Here's how the part is built. I have some questions about the finished solid (model axes, mm). A direction names the side the tool comes from. Round coordinates to 2 decimals unless told otherwise and drop trailing zeros. Order: outer loops, then holes, each group sorted by start corner. A loop starts at its lowest first (then second) coordinate and runs counter-clockwise, first axis right, second up. Notation, with made-up numbers: M 2.25,42 L 59.25,42 A22 ccw 59.25,72 Z; hole C 48.25,41 d11. An arc over 180 degrees is marked long. Write item = value, one per line. Start each with the question number.
Item 1: I want a section at A-A, the plane z = 0. List the corners of the cut face in (x, y) for me, plus the area to 3 significant figures.
Item 2: Please list where these lines run through material, in increasing order: L1, parallel to Y at x = 4.5, z = -1; L2, parallel to X at y = 1.5, z = 1.2; L3, parallel to X at y = -0.2, z = 1.6.
Item 3: I want a section at C-C, the plane x = 10. List the corners of the cut face in (y, z) for me.
Item 4: For faces 1 (the face through (1.5, 1, -1)), 2 (the face through (0.13, -2.13, 0.04)), which set-ups out of +Z, -Z, +X, -X, +Y, -Y let a thin tool reach every point of the face, with its end or its side?
Item 5: I want a section at B-B, the plane y = 0. List the corners of the cut face in (x, z) for me, plus the area to 3 significant figures.
Item 6: I'm going to push flat-ended pins straight in: P1, Ø1.5, axis at y = 0.5, z = 1.5, coming from the +X side; P2, Ø1.5, axis at x = 9, y = -1.5, coming from the +Z side; P3, Ø1.5, axis at x = 6.5, z = 0.5, coming from the +Y side. Where does each tip first touch, or does it pass through?
Autodesk Inventor part; units mm, degrees
ref_plane "YZ-Ebene" through (0, 0, 0) normal (1, 0, 0) x (0, 1, 0)
ref_plane "XZ-Ebene" through (0, 0, 0) normal (0, 1, 0) x (-1, 0, 0)
ref_plane "XY-Ebene" through (0, 0, 0) normal (0, 0, 1) x (1, 0, 0)
sketch "Skizze1" plane through (0, 0, 0) normal (0, 0, 1) x (1, 0, 0)
  line L0 (-2.3, 0) -> (13.8, 0)
  line L1 (0, -0.45) -> (0, 2.7)
  line L2 (0, 2.25) -> (1.5, 2.25)
  line L3 (1.5, 2.25) -> (1.5, 1.25)
  line L4 (1.5, 1.25) -> (11.5, 1.25)
  line L5 (11.5, 1.25) -> (11.5, 0)
  point P0 (0, 0)
  dimension "d0" = 1.5
  dimension "d1" = 10
  dimension "d16" = 2.5
  dimension "d17" = 4.5
revolve "Umdrehung1" add sketch "Skizze1" angle 360 about axis through (-10, 0, 0) along (1, 0, 0)
sketch "Skizze2" plane through (0, 0, 0) normal (-1, 0, 0) x (0, 0, 1)
  circle A0 centre (0, 0) radius 2.25
  line L0 (-3.15, 0) -> (3.15, 0)
  line L1 (2.2299, 0.3) -> (-2.2299, 0.3)
  line L2 (-2.2299, -0.3) -> (2.2299, -0.3)
  dimension "d5" = 0.6
extrude "Extrusion1" cut sketch "Skizze2" against normal blind 0.8 contours L0 A0 L1 | A0 L2 L0
chamfer "Fase1" distance 0.5 angle 45 1 edges at (11.5, -1.25, 0)
thread "Gewinde1"
chamfer "Fase2" distance 0.25 angle 45 3 edges at (0, -2.25, 0) (0, 1.6937, 1.4811) (0, 1.6937, -1.4811)
properties part number "Schlitzschraube_ra8846s-01" material "Stahl"
Filled in:
q1.outline = M 0,-2 L 0.25,-2.25 L 1.5,-2.25 L 1.5,-1.25 L 11,-1.25 L 11.5,-0.75 L 11.5,0.75 L 11,1.25 L 1.5,1.25 L 1.5,2.25 L 0.25,2.25 L 0,2 L 0,0.3 L 0.8,0.3 L 0.8,-0.3 L 0,-0.3 Z
q1.area = 31.0 mm^2
q2.L1 = -0.75 to 0.75
q2.L2 = 0 to 1.5
q2.L3 = 0.8 to 1.5
q3.outline = C 0,0 d2.5
q4.face_1 = +X
q4.face_2 = -X, -Y
q5.outline = M 0.8,-2.25 L 1.5,-2.25 L 1.5,-1.25 L 11,-1.25 L 11.5,-0.75 L 11.5,0.75 L 11,1.25 L 1.5,1.25 L 1.5,2.25 L 0.8,2.25 Z
q5.area = 27.9 mm^2
q6.P1 = 11.42
q6.P2 = 1
q6.P3 = 1.25
